Can you work these out from the model? Positions are in its coordinate system, mm. Coordinates: 2 decimals unless noted, no trailing zeros. Loops run counter-clockwise (first coordinate to the right, second up) from the corner with the lowest first, then second, coordinate; pieces in that order, holes last. Notation, with made-up numbers: (56.25, 18.25) -> (96.25, 18.25) arc R23 cw to (96.25, 42.25) -> close; hole circle Ø1 at (10, 43). An arc over 180 degrees is marked (long way). Use one line per item in the form item = value. Start each with the question number.
(1) I need wall thicknesses on line 1 (X direction, y = 0.2, z = 22). Which ranges of the line are inside material? Lowest first, please. Write a range as [from, to].
(2) I'm going to push flat-ended pins straight in: pin 1 (3 mm diameter, centred on x = -48.85, z = 79.25, fed in from -Y); pin 2 (1 mm diameter, centred on y = 0.5, z = 11, fed in from +X); pin 3 (1 mm diameter, centred on y = 0.5, z = 38.5, fed in from -X). Where does each tip first touch, or does it pass through?
(3) Imagine slicing it at A-A (y = 1.4). State how many separate pieces and enclosed holes the cut face has, plus the area to 3 significant figures.
(4) Imagine slicing it at B-B (z = 32). List the corners of the cut face in (x, y) for me, plus the area to 3 significant figures.
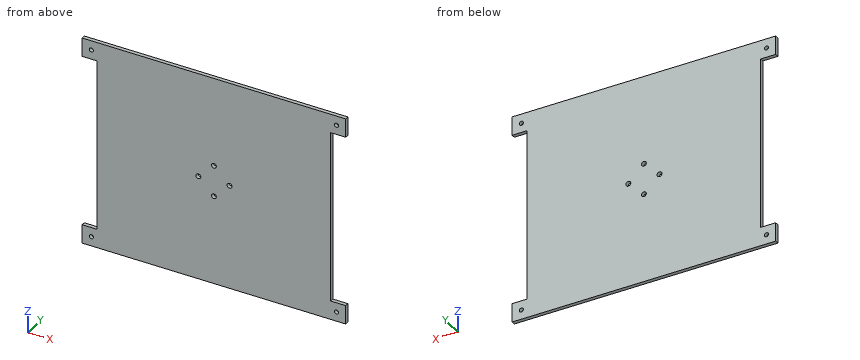
```python
from build123d import *

# Parameters (mm, degrees)
BOSS_EXTRUDE1_DEPTH = 2
SKETCH2_R           = 1.1
CUT_EXTRUDE1_DEPTH  = 2
SKETCH3_R           = 1.3
CUT_EXTRUDE2_DEPTH  = 2


with BuildPart() as part:
    # Sketch1 → Boss-Extrude1 (new body)
    with BuildSketch(Plane(origin=(0, 0, 0), x_dir=(1, 0, 0), z_dir=(0, 1, 0))):
        Polygon((-53.749139255, 17.446368981), (-45.749139255, 17.446368981), (-45.749139255, -74.253631019), (-53.749139255, -74.253631019), (-53.749139255, -84.253631019), (86.650860745, -84.253631019), (86.650860745, -74.253631019), (78.650860745, -74.253631019), (78.650860745, 17.446368981), (86.650860745, 17.446368981), (86.650860745, 27.446368981), (-53.749139255, 27.446368981), align=None)
    extrude(amount=BOSS_EXTRUDE1_DEPTH)

    # Sketch2 → Cut-Extrude1 (cut)
    with BuildSketch(Plane(origin=(0, 2, 0), x_dir=(1, 0, 0), z_dir=(0, 1, 0))):
        with Locations((-48.849139255, -79.253631019)):
            Circle(SKETCH2_R)
        with Locations((-48.849139255, 22.446368981)):
            Circle(SKETCH2_R)
        with Locations((81.750860745, 22.446368981)):
            Circle(SKETCH2_R)
        with Locations((81.750860745, -79.253631019)):
            Circle(SKETCH2_R)
    extrude(amount=-CUT_EXTRUDE1_DEPTH, mode=Mode.SUBTRACT)

    # Sketch3 → Cut-Extrude2 (cut)
    with BuildSketch(Plane(origin=(0, 2, 0), x_dir=(1, 0, 0), z_dir=(0, 1, 0))):
        with Locations((8.150860745, -28.403631019)):
            Circle(SKETCH3_R)
        with Locations((16.450860745, -36.703631019)):
            Circle(SKETCH3_R)
        with Locations((24.750860745, -28.403631019)):
            Circle(SKETCH3_R)
        with Locations((16.450860745, -20.103631019)):
            Circle(SKETCH3_R)
    extrude(amount=-CUT_EXTRUDE2_DEPTH, mode=Mode.SUBTRACT)


solid = part.part
```
Worked out:
q1.line_1 = [-45.75, 78.65]
q2.pin_1 = 0
q2.pin_2 = 78.65
q2.pin_3 = -45.75
q3.separate_pieces = 1
q3.enclosed_holes = 8
q3.area = 14,200 mm2
q4.outline = (-45.75, 0) -> (78.65, 0) -> (78.65, 2) -> (-45.75, 2) -> close
q4.area = 249 mm2
